```python
from build123d import *

# Parameters (mm, degrees)
F0_R      = 228.6
F1_DEPTH  = 381
F2_R      = 101.6
F3_DEPTH  = 114.3
F4_R      = 101.6
F3_FACE_R = 101.6
F5_DEPTH  = 114.3
F6_R      = 76.2
F7_DEPTH  = 25.4
F8_R      = 101.6
F9_DEPTH  = 50.8
F10_R     = 76.2
F11_DEPTH = 25.4
F12_R     = 101.6
F13_DEPTH = 50.8
F14_SIZE2 = 12.7
F14_SIZE  = 12.7


with BuildPart() as f1:
    # F0 (on Front) → F1 (new body)
    with BuildSketch(Plane.XZ):
        Circle(F0_R)
    extrude(amount=F1_DEPTH)

    # F2 (on face) → F3 (join)
    with BuildSketch(Plane.XZ.offset(381)):
        Circle(F2_R)
    extrude(amount=F3_DEPTH)

    # F4 (on face) + F3_face (on face) → F5 (join)
    with BuildSketch(Plane(origin=(0, 0, 0), x_dir=(-1, 0, 0), z_dir=(0, 1, 0))):
        Circle(F4_R)
    with BuildSketch(Plane.XZ.offset(495.3)):
        Circle(F3_FACE_R)
    extrude(amount=F5_DEPTH, dir=(0, 1, 0))

    # F6 (on face) → F7 (join)
    with BuildSketch(Plane(origin=(0, 114.3, 0), x_dir=(-1, 0, 0), z_dir=(0, 1, 0))):
        Circle(F6_R)
    extrude(amount=F7_DEPTH)

    # F8 (on face) → F9 (join)
    with BuildSketch(Plane(origin=(0, 139.7, 0), x_dir=(-1, 0, 0), z_dir=(0, 1, 0))):
        Circle(F8_R)
    extrude(amount=F9_DEPTH)

    # F10 (on face) → F11 (join)
    with BuildSketch(Plane.XZ.offset(495.3)):
        Circle(F10_R)
    extrude(amount=F11_DEPTH)

    # F12 (on face) → F13 (join)
    with BuildSketch(Plane.XZ.offset(520.7)):
        Circle(F12_R)
    extrude(amount=F13_DEPTH)

    # F14
    f14_edges = [f1.edges().sort_by_distance(p)[0] for p in [
        (101.6, 190.5, 0),
        (-101.6, -571.5, 0),
    ]]
    chamfer(f14_edges, length=F14_SIZE, length2=F14_SIZE2)


solid = f1.part
```
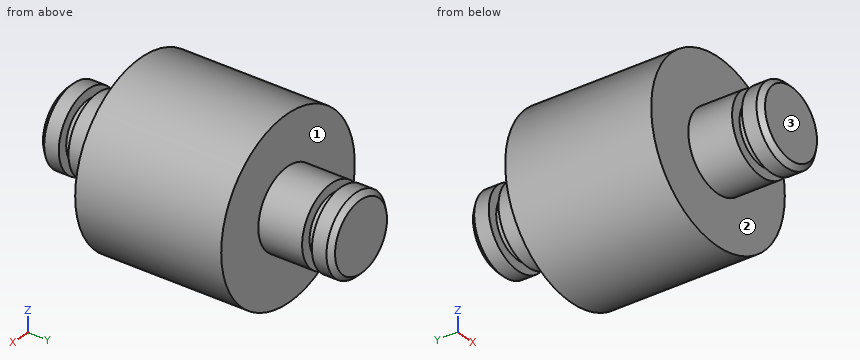
The model under review builds one solid part; all positions refer to its coordinate system, in mm. Face numbers are marked on the shaded views. A direction names the side the tool comes from. Coordinates: 2 decimals unless noted, no trailing zeros. Write each loop counter-clockwise with the first axis right and the second up, starting at its lowest first coordinate (ties: lowest second). Pieces come first, ordered by that corner, then holes. Notation, with made-up numbers: (23.5, 25.5) - (49.5, 25.5) arc R24 ccw to (49.5, 64.5) - close; hole circle Ø3 at (-6, -14.5). An arc over 180 degrees is marked (long way). Answer in a Markdown table with one row per item. Add a question column.
Q1. For the marked faces 1, 2 and 3, list the 3-axis set-ups (+Z, -Z, +X, -X, +Y, -Y) from which the entire face can be reached by the end or side of a thin tool; tool diameter is ignored.
Q2. Consider section C-C on y = -506. Give the boundary of the cut face in (x, z).
Q3. To check wall thickness, follow line 1 along Y through (x, z) = (-20.5, -84.5); line 2 along Y through (x, z) = (-206, -1); line 3 along Z through (x, y) = (-54, -2.5). State the ranges of each line that lie inside material, in increasing order. Write a range as from..to.
Q4. Clearance check with flat-ended pins moving along their axes: pin 1 (1 mm diameter, centred on x = 124, z = 6.5, fed in from -Y); pin 2 (4 mm diameter, centred on x = 113.5, y = -209.5, fed in from +Z); pin 3 (6 mm diameter, centred on x = -163, y = -90.5, fed in from -Z). State where each tip first meets the part, or that it passes through.
Q5. Consider section D-D on y = -410.5. Give the boundary of the cut face in (x, z), then the cut area to 3 significant figures.
Answers below:
| question | item | result |
|---|---|---|
| 1 | face 1 | +Y |
| 1 | face 2 | -Y |
| 1 | face 3 | +Z, -Z, +X, -X, -Y |
| 2 | outline | circle Ø152.4 at (0, 0) |
| 3 | line 1 | -571.5..-520.7, -495.3..114.3, 139.7..190.5 |
| 3 | line 2 | -381..0 |
| 3 | line 3 | -222.13..222.13 |
| 4 | pin 1 | y = -381 |
| 4 | pin 2 | z = 199.56 |
| 4 | pin 3 | z = -163.27 |
| 5 | outline | circle Ø203.2 at (0, 0) |
| 5 | area | 32,400 mm² |
